```python
from build123d import *

# Parameters (mm, degrees)
RESSALTO_EXTRUS_O1_DEPTH = 142.5
CORTE_EXTRUS_O1_DEPTH    = 50


with BuildPart() as part:
    # Esboço1 → Ressalto-extrusão1 (new, symmetric)
    with BuildSketch(Plane.XY):
        Polygon((0, 20), (0, -20), (20, -20), (20, -18.5), (1.5, -18.5), (1.5, 18.5), (20, 18.5), (20, 20), align=None)
    extrude(amount=RESSALTO_EXTRUS_O1_DEPTH, both=True)

    # Esboço2 → Corte-extrusão1 (cut, symmetric)
    with BuildSketch(Plane(origin=(0, 20, 0), x_dir=(1, 0, 0), z_dir=(0, 1, 0))):
        Polygon((1.5, -142.5), (20, -124), (20, -142.5), align=None)
        Polygon((0, 142.5), (20, 122.5), (20, 142.5), align=None)
    extrude(amount=CORTE_EXTRUS_O1_DEPTH, both=True, mode=Mode.SUBTRACT)


solid = part.part
```
Geometry check sheet. Reference: the model listing, model coordinates, mm. A direction names the side the tool comes from. Coordinates: 2 decimals unless noted, no trailing zeros. Order: outer loops, then holes, each group sorted by start corner. A loop starts at its lowest first (then second) coordinate and runs counter-clockwise, first axis right, second up.
Item 1: Section check C-C (z = 91). Enter the section's corners in (x, y), plus the area to 4 significant figures.
Item 2: Section check D-D (y = 13.5). Enter the section's corners in (x, z), plus the area to 3 significant figures.
Item 3: Section check B-B (x = 16). Enter the section's corners in (y, z).
Item 4: Section check A-A (x = 5.25). Enter the section's corners in (y, z).
Item 5: Depth check by flat-ended pin: pin 1 (1 mm diameter, centred on y = 8.5, z = -49.5, fed in from +X); pin 2 (1.5 mm diameter, centred on x = 4, y = -14, fed in from +Z). Enter the tip coordinate at first touch or a pass-through.
Item 6: Mould release check, pull along Y, two halves, no side actions. Record for faces 3 (the flat face through (10, 20, 2)), 4 (the flat face through (11, -18.5, 3)), 5 (the flat face through (11, -19, 133)): released by +Y, released by -Y, zero draft, split by the parting line, or undercut.
Item 7: Scan lines: line 1 along Y through (x, z) = (15.25, -44); line 2 along X through (y, z) = (4.5, -130). Record each from-to range of solid material in increasing order.
Item 8: Tool access check on faces 1 (the flat face through (11, 19, 133)), 2 (the flat face through (1.5, 0, 3)). Record the directions out of +Z, -Z, +X, -X, +Y, -Y that give a thin tool (end or side, any length) a straight path to the whole face; none if there is none.
Check sheet entries:
1. outline: (0, -20) - (20, -20) - (20, -18.5) - (1.5, -18.5) - (1.5, 18.5) - (20, 18.5) - (20, 20) - (0, 20) - close
1. area: 115.5 mm2
2. outline: (0, -142.5) - (1.5, -141) - (1.5, 142.5) - (0, 142.5) - close
2. area: 426 mm2
3. outline: (-20, -126.5) - (-18.5, -126.5) - (-18.5, 128) - (-20, 128) - close; (18.5, -126.5) - (20, -126.5) - (20, 128) - (18.5, 128) - close
4. outline: (-20, -137.25) - (-18.5, -137.25) - (-18.5, 138.75) - (-20, 138.75) - close; (18.5, -137.25) - (20, -137.25) - (20, 138.75) - (18.5, 138.75) - close
5. pin 1: stops at x = 1.5
5. pin 2: passes through
6. face 3: released by +Y
6. face 4: undercut
6. face 5: zero draft
7. line 1: y = -20 to -18.5, 18.5 to 20
7. line 2: x = 0 to 1.5
8. face 1: +Z, +X, +Y, -Y
8. face 2: +Z, -Z, +X
